from build123d import *

# Parameters (mm, degrees)
BOSS_EXTRUDE1_DEPTH        = 9
F_12_0MM_DOWEL_HOLE1_D     = 12
F_12_0MM_DOWEL_HOLE1_DEPTH = 18
F_12_0MM_DOWEL_HOLE1_TIP   = 4.047051101
SKETCH6_R                  = 3
CUT_EXTRUDE1_DEPTH         = 50.244289009
CHAMFER1_SIZE              = 2


with BuildPart() as part:
    # Sketch1 → Boss-Extrude1 (new, symmetric)
    with BuildSketch(Plane.XY):
        Polygon((-19, 30), (19, 30), (19, -30), (13.75, -30), (13.75, -27.5), (11.25, -27.5), (11.25, -25), (8.75, -25), (8.75, -22.5), (6.25, -22.5), (6.25, -20), (3.75, -20), (3.75, -17.5), (1.25, -17.5), (1.25, -15), (-1.25, -15), (-1.25, -17.5), (-3.75, -17.5), (-3.75, -20), (-6.25, -20), (-6.25, -22.5), (-8.75, -22.5), (-8.75, -25), (-11.25, -25), (-11.25, -27.5), (-13.75, -27.5), (-13.75, -30), (-19, -30), align=None)
    extrude(amount=BOSS_EXTRUDE1_DEPTH, both=True)

    # Ø12.0mm Dowel Hole1
    with Locations(Plane(origin=(-0.020341947, 30, -0.020341947), x_dir=(1, 0, 0), z_dir=(0, 1, 0))):
        with Locations((0, 0)):
            Hole(F_12_0MM_DOWEL_HOLE1_D / 2, depth=F_12_0MM_DOWEL_HOLE1_DEPTH)
            with Locations((0, 0, -(F_12_0MM_DOWEL_HOLE1_DEPTH + F_12_0MM_DOWEL_HOLE1_TIP / 2))):  # 112° drill point
                Cone(0, F_12_0MM_DOWEL_HOLE1_D / 2, F_12_0MM_DOWEL_HOLE1_TIP, mode=Mode.SUBTRACT)

    # Sketch6 → Cut-Extrude1 (cut, through all)
    with BuildSketch(Plane.ZY.offset(19)):
        with Locations((0, 23)):
            Circle(SKETCH6_R)
    extrude(amount=-CUT_EXTRUDE1_DEPTH, mode=Mode.SUBTRACT)

    # Chamfer1
    chamfer1_edges = [part.edges().sort_by_distance(p)[0] for p in [
        (0, 30, 9),
        (0, 30, -9),
        (-19, 30, 0),
        (19, 30, 0),
    ]]
    chamfer(chamfer1_edges, length=CHAMFER1_SIZE)


solid = part.part
Build history of the part. All positions in model axes, mm. A direction names the side the tool comes from. Round coordinates to 2 decimals unless told otherwise and drop trailing zeros. Loops run counter-clockwise (first coordinate to the right, second up) from the corner with the lowest first, then second, coordinate; pieces in that order, holes last. Notation, with made-up numbers: (65, -12) -> (116, -12) arc R12 cw to (116, 10) -> close; hole circle Ø4 at (47, 52). An arc over 180 degrees is marked (long way). Answer in a Markdown table with one row per item.
Item 1: Mould opens along Z. For faces 1 (the cylindrical face through (4.74, 20.87, 3.63)), 2 (the flat face through (-11.25, -26, 0)), 3 (the flat face through (0, -1, -9)) say: +Z half, -Z half, draft (parallel to the pull), parting line (faces both ways), or undercut.
Answers below:
| item | result |
|---|---|
| face 1 | undercut |
| face 2 | draft |
| face 3 | -Z half |
Item 2: Saw through at B-B (y = 18). Write the cut outline in (x, z), and give its area (3 significant figures).
Answers below:
| item | result |
|---|---|
| outline | (-19, -9) -> (19, -9) -> (19, 9) -> (-19, 9) -> close; hole circle Ø12 at (-0.02, -0.02) |
| area | 571 mm² |
Item 3: Pin check, flat tips, straight feed: pin 1 (0.8 mm diameter, centred on x = -12.5, z = 3.5, fed in from -Y); pin 2 (3 mm diameter, centred on x = 0, z = -4, fed in from -Y); pin 3 (3 mm diameter, centred on x = 9.5, z = 4, fed in from -Y). Stop position of each tip, or through.
Answers below:
| item | result |
|---|---|
| pin 1 | stops at y = -27.5 |
| pin 2 | stops at y = -17.5 |
| pin 3 | stops at y = -25 |
Item 4: Saw through at A-A (y = -21.5). Write the cut outline in (x, z).
Answers below:
| item | result |
|---|---|
| outline | (-19, -9) -> (-6.25, -9) -> (-6.25, 9) -> (-19, 9) -> close; (6.25, -9) -> (19, -9) -> (19, 9) -> (6.25, 9) -> close |
Item 5: Which spindle directions (+Z, -Z, +X, -X, +Y, -Y) get a long thin tool onto all of the face, cutting with end or side? Do faces 4 (the flat face through (5, -20, 0)), 5 (the flat face through (0, 29, -8)). Say none if no direction does.
Answers below:
| item | result |
|---|---|
| face 4 | +Z, -Z, -Y |
| face 5 | -Z, +X, -X, +Y |
Item 6: Drill centre lines: L1, parallel to Z at x = -15, y = 23; L2, parallel to X at y = -16, z = -2.25; L3, parallel to Y at x = -9.75, z = 0. Where is each one in solid material? Low to high. Write a range as [from, to].
Answers below:
| item | result |
|---|---|
| L1 | z = [-9, -3], [3, 9] |
| L2 | x = [-19, -1.25], [1.25, 19] |
| L3 | y = [-25, 20], [26, 30] |
